from build123d import *

# Parameters (mm, degrees)
BOSS_EXTRUDE1_DEPTH = 16
CUT_EXTRUDE1_REACH  = 41.786
SKETCH4_R           = 1.5875
CUT_EXTRUDE2_REACH  = 41.786
SKETCH5_R           = 2.159
FILLET1_R           = 2


with BuildPart() as part:
    # Sketch1 → Boss-Extrude1 (new body)
    with BuildSketch(Plane(origin=(0, 0, 0), x_dir=(1, 0, 0), z_dir=(0, 1, 0))):
        with BuildLine():
            Line((1, -16.469669092), (1.512240508, -24.90610075))
            Line((1.512240508, -24.90610075), (7.512240508, -24.90610075))
            Line((7.512240508, -24.90610075), (7.512240508, -16.90610075))
            ThreePointArc((7.512240508, -16.90610075), (18.445940235, -1.413254699), (10, 15.564382416))
            Line((10, 15.564382416), (10, 25.5))
            Line((10, 25.5), (-10, 25.5))
            Line((-10, 25.5), (-10, 15.564382416))
            ThreePointArc((-10, 15.564382416), (-18.445940235, -1.413254699), (-7.512240508, -16.90610075))
            Line((-7.512240508, -16.90610075), (-7.512240508, -24.90610075))
            Line((-7.512240508, -24.90610075), (-1.512240508, -24.90610075))
            Line((-1.512240508, -24.90610075), (-1, -16.469669092))
            ThreePointArc((-1, -16.469669092), (0, 16.5), (1, -16.469669092))
        make_face()
    extrude(amount=BOSS_EXTRUDE1_DEPTH)

    # Cut-Sweep1: sweep along a path in Sketch2
    with BuildLine(Plane(origin=(0, 0, 0), x_dir=(0, 0, -1), z_dir=(1, 0, 0))) as cut_sweep1_path:
        Line((19.5, 11.510254581), (21.5, 0))
    # Sketch3 → Cut-Sweep1 (sweep, cut)
    with BuildSketch(Plane(origin=(0, 0, 0), x_dir=(1, 0, 0), z_dir=(0, 1, 0))):
        with BuildLine():
            Line((-7.5, 20.14944168), (-7.5, 12.323332295))
            Line((-7.5, 12.323332295), (7.5, 12.323332295))
            Line((7.5, 12.323332295), (7.5, 20.14944168))
            ThreePointArc((7.5, 20.14944168), (0, 21.5), (-7.5, 20.14944168))
        make_face()
    sweep(path=cut_sweep1_path.line, mode=Mode.SUBTRACT)

    # Cut-Extrude1: up to this plane
    cut_extrude1_end = Plane(origin=(-1, 16, 16.469669092), z_dir=(-0.9981617631515517, 0, -0.06060606060606122))
    # Sketch4 → Cut-Extrude1 (cut, up to the surface)
    with BuildSketch(Plane.ZY.offset(7.512240508), mode=Mode.PRIVATE) as cut_extrude1_sk1:
        with Locations((20.90610075, 8)):
            Circle(SKETCH4_R)
    cut_extrude1_tool1 = split(extrude(cut_extrude1_sk1.sketch, amount=-CUT_EXTRUDE1_REACH, mode=Mode.PRIVATE), bisect_by=cut_extrude1_end, keep=Keep.BOTH, mode=Mode.PRIVATE)
    add(cut_extrude1_tool1.solids().sort_by_distance((-7.512241, 8, 20.906101))[0], mode=Mode.SUBTRACT)

    # Cut-Extrude2: up to this plane
    cut_extrude2_end = Plane(origin=(1, 16, 16.469669092), z_dir=(0.9981617631515518, 0, -0.06060606060606071))
    # Sketch5 → Cut-Extrude2 (cut, up to the surface)
    with BuildSketch(Plane(origin=(7.512240508, 0, 0), x_dir=(0, 0, -1), z_dir=(1, 0, 0)), mode=Mode.PRIVATE) as cut_extrude2_sk1:
        with Locations((-20.90610075, 8)):
            Circle(SKETCH5_R)
    cut_extrude2_tool1 = split(extrude(cut_extrude2_sk1.sketch, amount=-CUT_EXTRUDE2_REACH, mode=Mode.PRIVATE), bisect_by=cut_extrude2_end, keep=Keep.BOTH, mode=Mode.PRIVATE)
    add(cut_extrude2_tool1.solids().sort_by_distance((7.512241, 8, 20.906101))[0], mode=Mode.SUBTRACT)

    # Fillet1
    fillet1_edges = [part.edges().sort_by_distance(p)[0] for p in [
        (-10, 8, -25.5),
        (10, 8, -25.5),
    ]]
    fillet(fillet1_edges, radius=FILLET1_R)


solid = part.part
Source: CAD feature listing. Evaluate the final solid. Frame: model axes, mm. A direction names the side the tool comes from. Round coordinates to 2 decimals unless told otherwise and drop trailing zeros. Loops run counter-clockwise (first coordinate to the right, second up) from the corner with the lowest first, then second, coordinate; pieces in that order, holes last. Notation, with made-up numbers: M -15,75.5 L 39,75.5 A11 cw 39,91.5 Z; hole C 74,-7.5 d1. An arc over 180 degrees is marked long. Return JSON: item names as keys, results as strings. Group by question number.
1. Section query C-C on x = -6. State how many separate pieces and enclosed holes the cut face has, and give its area (3 significant figures).
2. Section query B-B on x = 15. Output: boundary loops of the cut face in (y, z), and give its area (3 significant figures).
3. Mould query, pull axis X, two halves, no side actions, for faces 1 (the face through (-10, 8, -20)), 2 (the face through (-1, 16, -17)), 3 (the face through (18.423, 7.888, 1.691)), 4 (the face through (7.5, 6, -17)). Classes: released by +X, released by -X, zero draft, split by the parting line, or undercut.
4. Reachability of faces 5 (the face through (4.4, 7.2, 18.9)), 6 (the face through (-1.26, 6.11, 20.75)), 7 (the face through (10, 8, -19)), 8 (the face through (-7.512, 8, 19)), 9 (the face through (7.512, 6, 19)) from +Z, -Z, +X, -X, +Y, -Y: full face, straight path, thin tool, end or side. Return the list, or none.
5. Pin query (flat end, axial travel): pin 1 (4 mm diameter, centred on y = 6.5, z = 22, fed in from -X); pin 2 (4 mm diameter, centred on y = 3, z = 8.5, fed in from -X); pin 3 (6 mm diameter, centred on y = 4, z = -18, fed in from +X); pin 4 (3 mm diameter, centred on y = 8, z = 20.91, fed in from +X). Return the tip coordinate at first contact, or that it passes through.
6. Material intervals for line 1 along X through (y, z) = (5, -17.5); line 2 along X through (y, z) = (9.25, 0); line 3 along Z through (x, y) = (4, 8), sorted ascending. Write a range as from..to.
7. Section query A-A on z = 0. Output: boundary loops of the cut face in (x, y), and give its area (3 significant figures).
Checks:
{
 "1": {"separate pieces": "2", "enclosed holes": "1", "area": "258 mm²"},
 "2": {"outline": "M 0,-10.83 L 16,-10.83 L 16,-6.87 L 0,-6.87 Z; M 0,6.87 L 16,6.87 L 16,10.83 L 0,10.83 Z", "area": "127 mm²"},
 "3": {"face 1": "released by -X", "face 2": "zero draft", "face 3": "released by +X", "face 4": "undercut"},
 "4": {"face 5": "+X", "face 6": "+Z, +Y, -Y", "face 7": "-Z, +X, +Y, -Y", "face 8": "+Z, -X, +Y, -Y", "face 9": "+Z, +X, +Y, -Y"},
 "5": {"pin 1": "stops at x = -7.51", "pin 2": "stops at x = -17.32", "pin 3": "stops at x = 10.83", "pin 4": "passes through"},
 "6": {"line 1": "x = -10..-7.5, 7.5..10", "line 2": "x = -18.5..-16.5, 16.5..18.5", "line 3": "z = -25.5..-19.73, 16.01..18.75, 23.07..24.91"},
 "7": {"outline": "M -18.5,0 L -16.5,0 L -16.5,16 L -18.5,16 Z; M 16.5,0 L 18.5,0 L 18.5,16 L 16.5,16 Z", "area": "64.0 mm²"}
}
